Design review of the part built by this model. Coordinates are the model's own, in mm. Face numbers are marked on the shaded views. A direction names the side the tool comes from. Coordinates: 2 decimals unless noted, no trailing zeros. Loops run counter-clockwise (first coordinate to the right, second up) from the corner with the lowest first, then second, coordinate; pieces in that order, holes last.
Q1. Machinability: for the marked faces 4, 5, 6, 7 and 8, which of the approach directions +Z, -Z, +X, -X, +Y, -Y give a long, thin tool a straight path to every point of the face, cutting with its end or side? Answer none if there is none.
Q2. Draft analysis for pull direction Y (two halves, no side actions). For the marked faces 1, 2 and 3, state which applies: released by +Y, released by -Y, zero draft, split by the parting line, or undercut.
Q3. Add section C-C on y = 10. Give the boundary of the cut face in (x, z) (3 decimals), and give its area (3 significant figures).
Q4. Wall thickness on probe 1 along Z at (x, y) = (12, 13.5); probe 2 along Y at (x, z) = (-9.5, -8.25); probe 3 along Y at (x, z) = (-3, -4): over which ranges is each line inside the solid? List them lowest first.
Q5. Add section A-A on z = -7.5. Give the boundary of the cut face in (x, y), and give its area (3 significant figures).
Q6. Add section D-D on x = -7.5. Give the boundary of the cut face in (y, z).
Q7. For P1, Ø6, axis at x = 14.5, y = -5, coming from the +Z side; P2, Ø2.5, axis at y = -1.5, z = -13.5, coming from the -X side; P3, Ø2.5, axis at x = -6, z = -14.5, coming from the +Y side; P4, Ø0.8, axis at x = -11, z = -13, coming from the +Y side, all flat-tipped, find the tip position at first contact; note any pin that passes through.
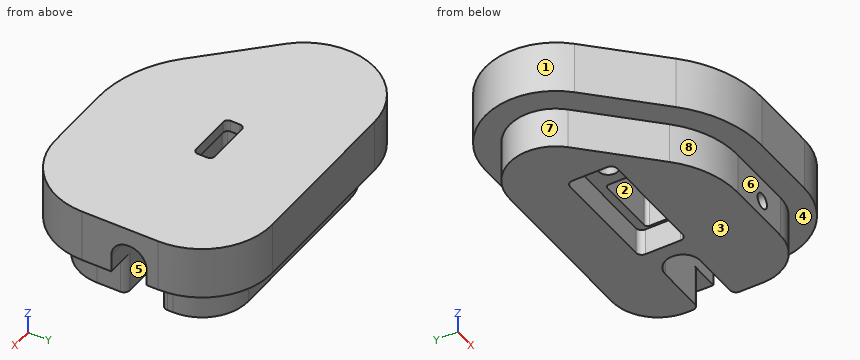
```python
from build123d import *

# Parameters (mm, degrees)
EXTRUDE_1_DEPTH     = 9
EXTRUDE_2_DEPTH     = 7
SKETCH_6_R          = 1.3
CUT_EXTRUDE_1_DEPTH = 6
SKETCH_7_R          = 1.3
CUT_EXTRUDE_2_DEPTH = 6
CUT_EXTRUDE_3_DEPTH = 14
CUT_EXTRUDE_4_DEPTH = 2
EXTRUDE_START       = 9.4
EXTRUDE_4_DEPTH     = 9.4
SKETCH_11_R         = 1.3
CUT_EXTRUDE_5_DEPTH = 6
CHAMFER_1_SIZE      = 0.4
CHAMFER_1_SIZE2     = 1.098990968
CUT_EXTRUDE_6_DEPTH = 13
FILLET_1_R          = 3
FILLET_2_R          = 1


with BuildPart() as part:
    # 草图2 → 凸台-拉伸1 (new body)
    with BuildSketch(Plane.XY):
        with BuildLine():
            Line((-24.798989873, -3.485281374), (-14.142135624, -14.142135624))
            ThreePointArc((-14.142135624, -14.142135624), (-7.653668647, -18.47759065), (0, -20))
            Line((0, -20), (11.686291501, -20))
            ThreePointArc((11.686291501, -20), (20.171572875, -16.485281374), (23.686291501, -8))
            Line((23.686291501, -8), (23.686291501, 5))
            ThreePointArc((23.686291501, 5), (20.171572875, 13.485281374), (11.686291501, 17))
            Line((11.686291501, 17), (-16.313708499, 17))
            ThreePointArc((-16.313708499, 17), (-27.400262889, 9.592201188), (-24.798989873, -3.485281374))
        make_face()
    extrude(amount=-EXTRUDE_1_DEPTH)

    # 草图3 → 凸台-拉伸2 (add)
    with BuildSketch(Plane(origin=(0, 0, -9), x_dir=(-1, 0, 0), z_dir=(0, 0, -1))):
        with BuildLine():
            Line((16.313708499, 12.9), (-11.686291501, 12.9))
            ThreePointArc((-11.686291501, 12.9), (-17.272435072, 10.586143571), (-19.586291501, 5))
            Line((-19.586291501, 5), (-19.586291501, -8))
            ThreePointArc((-19.586291501, -8), (-17.272435072, -13.586143571), (-11.686291501, -15.9))
            Line((-11.686291501, -15.9), (0, -15.9))
            ThreePointArc((0, -15.9), (6.084666575, -14.689684567), (11.242997821, -11.242997821))
            Line((11.242997821, -11.242997821), (21.89985207, -0.586143571))
            ThreePointArc((21.89985207, -0.586143571), (23.612356806, 8.023199116), (16.313708499, 12.9))
        make_face()
    extrude(amount=EXTRUDE_2_DEPTH)

    # 草图6 → 切除-拉伸1 (cut)
    with BuildSketch(Plane(origin=(0, 12.9, 0), x_dir=(1, 0, 0), z_dir=(0, 1, 0))):
        with Locations(Location((-11.313708499, 13, 0), (0, 0, 180))):
            Circle(SKETCH_6_R)
    extrude(amount=-CUT_EXTRUDE_1_DEPTH, mode=Mode.SUBTRACT)

    # 草图7 → 切除-拉伸2 (cut)
    with BuildSketch(Plane.XZ.offset(15.9)):
        with Locations(Location((6.686291501, -13, 0), (0, 0, 270))):
            Circle(SKETCH_7_R)
    extrude(amount=-CUT_EXTRUDE_2_DEPTH, mode=Mode.SUBTRACT)

    # 草图8 → 切除-拉伸3 (cut)
    with BuildSketch(Plane(origin=(0, 0, -16), x_dir=(-1, 0, 0), z_dir=(0, 0, -1))):
        with BuildLine():
            Line((-4, 4), (14, 4))
            ThreePointArc((14, 4), (14.707106781, 3.707106781), (15, 3))
            Line((15, 3), (15, -3))
            ThreePointArc((15, -3), (14.707106781, -3.707106781), (14, -4))
            Line((14, -4), (-4, -4))
            ThreePointArc((-4, -4), (-4.707106781, -3.707106781), (-5, -3))
            Line((-5, -3), (-5, 3))
            ThreePointArc((-5, 3), (-4.707106781, 3.707106781), (-4, 4))
        make_face()
    extrude(amount=-CUT_EXTRUDE_3_DEPTH, mode=Mode.SUBTRACT)

    # 草图9 → 切除-拉伸4 (cut)
    with BuildSketch(Plane(origin=(0, 0, -2), x_dir=(-1, 0, 0), z_dir=(0, 0, -1))):
        with BuildLine():
            Line((-2.7, 1.6), (4.7, 1.6))
            ThreePointArc((4.7, 1.6), (5.265685425, 1.365685425), (5.5, 0.8))
            Line((5.5, 0.8), (5.5, -0.8))
            ThreePointArc((5.5, -0.8), (5.265685425, -1.365685425), (4.7, -1.6))
            Line((4.7, -1.6), (-2.7, -1.6))
            ThreePointArc((-2.7, -1.6), (-3.265685425, -1.365685425), (-3.5, -0.8))
            Line((-3.5, -0.8), (-3.5, 0.8))
            ThreePointArc((-3.5, 0.8), (-3.265685425, 1.365685425), (-2.7, 1.6))
        make_face()
    extrude(amount=-CUT_EXTRUDE_4_DEPTH, mode=Mode.SUBTRACT)

    # 草图10 → 凸台-拉伸4 (add)
    with BuildSketch(Plane(origin=(0, 0, -2), x_dir=(-1, 0, 0), z_dir=(0, 0, -1)).offset(EXTRUDE_START)):
        with BuildLine():
            Line((14, 4), (-4, 4))
            ThreePointArc((-4, 4), (-4.707106781, 3.707106781), (-5, 3))
            Line((-5, 3), (-5, -3))
            ThreePointArc((-5, -3), (-4.707106781, -3.707106781), (-4, -4))
            Line((-4, -4), (14, -4))
            ThreePointArc((14, -4), (14.707106781, -3.707106781), (15, -3))
            Line((15, -3), (15, 3))
            ThreePointArc((15, 3), (14.707106781, 3.707106781), (14, 4))
        make_face()
        with BuildLine():
            Line((-4, -2.6), (6, -2.6))
            ThreePointArc((6, -2.6), (6.424264069, -2.424264069), (6.6, -2))
            Line((6.6, -2), (6.6, 2))
            ThreePointArc((6.6, 2), (6.424264069, 2.424264069), (6, 2.6))
            Line((6, 2.6), (-4, 2.6))
            ThreePointArc((-4, 2.6), (-4.424264069, 2.424264069), (-4.6, 2))
            Line((-4.6, 2), (-4.6, -2))
            ThreePointArc((-4.6, -2), (-4.424264069, -2.424264069), (-4, -2.6))
        make_face(mode=Mode.SUBTRACT)
    extrude(amount=-EXTRUDE_4_DEPTH)

    # 草图11 → 切除-拉伸5 (cut)
    with BuildSketch(Plane(origin=(0, 0, -11.4), x_dir=(-1, 0, 0), z_dir=(0, 0, -1))):
        with Locations((10, 0)):
            Circle(SKETCH_11_R)
    extrude(amount=-CUT_EXTRUDE_5_DEPTH, mode=Mode.SUBTRACT)

    # 倒角1
    chamfer_1_edges = [part.edges().sort_by_distance(p)[0] for p in [
        (-8.7, 0, -11.4),
    ]]
    chamfer_1_side = [part.faces().sort_by_distance(p)[0] for p in [
        (-7.139463972, 0, -11.4),
    ]]
    chamfer(chamfer_1_edges, length=CHAMFER_1_SIZE, length2=CHAMFER_1_SIZE2, reference=chamfer_1_side[0])

    # 草图14 → 切除-拉伸6 (cut)
    with BuildSketch(Plane(origin=(0, 0, -16), x_dir=(-1, 0, 0), z_dir=(0, 0, -1))):
        with BuildLine():
            Line((-10.5, 3), (-23.686291501, 3))
            Line((-23.686291501, 3), (-23.686291501, -3))
            Line((-23.686291501, -3), (-10.5, -3))
            ThreePointArc((-10.5, -3), (-7.5, 0), (-10.5, 3))
        make_face()
    extrude(amount=-CUT_EXTRUDE_6_DEPTH, mode=Mode.SUBTRACT)

    # 圆角1
    fillet_1_edges = [part.edges().sort_by_distance(p)[0] for p in [
        (17.093145751, -3, -3),
        (17.093145751, 3, -3),
        (7.5, 0, -3),
    ]]
    fillet(fillet_1_edges, radius=FILLET_1_R - 0.0001)  # a hair under: the kernel refuses the full size

    # 圆角2
    fillet_2_edges = [part.edges().sort_by_distance(p)[0] for p in [
        (19.586291501, 3, -12.5),
        (19.586291501, -3, -12.5),
    ]]
    fillet(fillet_2_edges, radius=FILLET_2_R)


solid = part.part
```
Entries:
1. face 4: -Z
1. face 5: -Z, +X
1. face 6: -Z, +X, -X, -Y
1. face 7: -Z, -X
1. face 8: -Z, -X, -Y
2. face 1: split by the parting line
2. face 2: undercut
2. face 3: zero draft
3. outline: (-27.222, -9) - (-22.43, -9) - (-22.43, -16) - (17.803, -16) - (17.803, -9) - (22.595, -9) - (22.595, 0) - (-27.222, 0) - close; hole circle Ø2.6 at (-11.314, -13)
3. area: 725 mm2
4. probe 1: z = -9 to 0
4. probe 2: y = -17.6 to -1.2, 1.2 to 17
4. probe 3: y = -19.77 to -2.6, 2.6 to 17
5. outline: (-24.8, -3.49) - (-14.14, -14.14) arc R20 ccw to (0, -20) - (11.69, -20) arc R12 ccw to (23.69, -8) - (23.69, -3) - (10.5, -3) arc R3 cw to (10.5, 3) - (23.69, 3) - (23.69, 5) arc R12 ccw to (11.69, 17) - (-16.31, 17) arc R12 ccw to start; hole circle Ø2.6 at (-10, 0); hole (-6.6, -2) arc R0.6 ccw to (-6, -2.6) - (4, -2.6) arc R0.6 ccw to (4.6, -2) - (4.6, 2) arc R0.6 ccw to (4, 2.6) - (-6, 2.6) arc R0.6 ccw to (-6.6, 2) - close
5. area: 1,460 mm2
6. outline: (-18.54, -9) - (-14.02, -9) - (-14.02, -16) - (-4, -16) - (-4, -11.4) - (4, -11.4) - (4, -16) - (12.9, -16) - (12.9, -9) - (17, -9) - (17, 0) - (-18.54, 0) - close
7. P1: stops at z = 0
7. P2: stops at x = -22.22
7. P3: stops at y = 12.9
7. P4: stops at y = 6.9
